Job drawing, mm, ordinate dimensions from the low corner. One solid piece. Coordinates: 2 decimals unless noted, no trailing zeros. Loops run counter-clockwise (first coordinate to the right, second up) from the corner with the lowest first, then second, coordinate; pieces in that order, holes last. Notation, with made-up numbers: M 14.5,28 L 35.5,28 A19 cw 35.5,33 Z; hole C 17.25,-3.5 d11. An arc over 180 degrees is marked long. Answer as a JSON object with one key per item and string values. Group by question number.
1. Saw through at A-A on z = 16.52. Write the cut outline in (x, y), then the cut area to 3 significant figures.
2. Saw through at B-B on x = 235.14. Write the cut outline in (y, z), then the cut area to 3 significant figures.
3. Drill centre lines: L1, parallel to X at y = 2.75, z = 48.48; L2, parallel to X at y = 2.75, z = 16.52; L3, parallel to Z at x = 288.48, y = 3.25. Where is each one in solid material? Low to high.
4. Saw through at D-D on x = 288.48. Write the cut outline in (y, z).
5. Saw through at C-C on z = 48.48. Write the cut outline in (x, y), then the cut area to 3 significant figures.
6. Drop a flat-ended pin along its axis: pin 1 Ø6 at (x, z) = (288.48, 48.48) entering from +Y. Give the stop position or say it passes through.
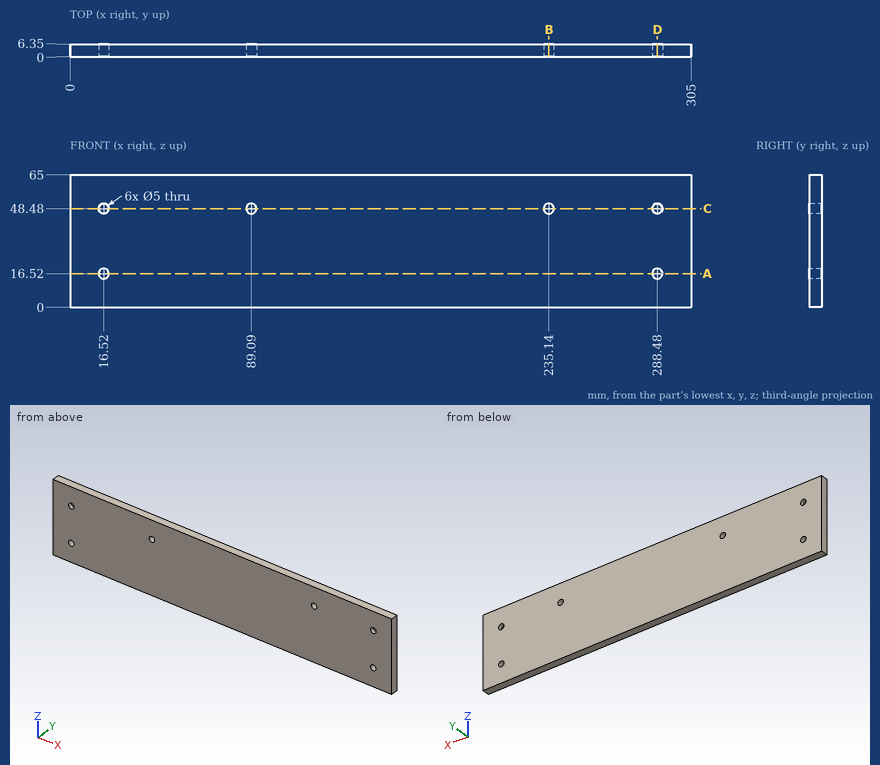
Outcome:
{
 "1": {"outline": "M 0,0 L 14.02,0 L 14.02,6.35 L 0,6.35 Z; M 19.02,0 L 285.98,0 L 285.98,6.35 L 19.02,6.35 Z; M 290.98,0 L 305,0 L 305,6.35 L 290.98,6.35 Z", "area": "1,870 mm²"},
 "2": {"outline": "M 0,0 L 6.35,0 L 6.35,45.98 L 0,45.98 Z; M 0,50.98 L 6.35,50.98 L 6.35,65 L 0,65 Z", "area": "381 mm²"},
 "3": {"L1": "x = 0 to 14.02, 19.02 to 86.59, 91.59 to 232.64, 237.64 to 285.98, 290.98 to 305", "L2": "x = 0 to 14.02, 19.02 to 285.98, 290.98 to 305", "L3": "z = 0 to 14.02, 19.02 to 45.98, 50.98 to 65"},
 "4": {"outline": "M 0,0 L 6.35,0 L 6.35,14.02 L 0,14.02 Z; M 0,19.02 L 6.35,19.02 L 6.35,45.98 L 0,45.98 Z; M 0,50.98 L 6.35,50.98 L 6.35,65 L 0,65 Z"},
 "5": {"outline": "M 0,0 L 14.02,0 L 14.02,6.35 L 0,6.35 Z; M 19.02,0 L 86.59,0 L 86.59,6.35 L 19.02,6.35 Z; M 91.59,0 L 232.64,0 L 232.64,6.35 L 91.59,6.35 Z; M 237.64,0 L 285.98,0 L 285.98,6.35 L 237.64,6.35 Z; M 290.98,0 L 305,0 L 305,6.35 L 290.98,6.35 Z", "area": "1,810 mm²"},
 "6": {"pin 1": "stops at y = 6.35"}
}
